Input: part model. Units: mm. Frame: model coordinates. A direction names the side the tool comes from. Round coordinates to 2 decimals unless told otherwise and drop trailing zeros. Write each loop counter-clockwise with the first axis right and the second up, starting at its lowest first coordinate (ties: lowest second). Pieces come first, ordered by that corner, then holes. Notation, with made-up numbers: (17.5, 40) - (39.5, 40) arc R13 cw to (39.5, 62) - close; hole circle Ø1 at (-15.75, 80.5). An arc over 180 degrees is marked (long way). One line per item, written item: value. Start each with the question number.
```python
from build123d import *

# Parameters (mm, degrees)
BOSS_EXTRUDE1_DEPTH = 4
CHAMFER1_SIZE       = 0.4
BOSS_EXTRUDE2_START = 4
SKETCH3_R           = 2.5
BOSS_EXTRUDE2_DEPTH = 0.01


with BuildPart() as part:
    # Sketch1 → Boss-Extrude1 (new body)
    with BuildSketch(Plane(origin=(0, 0, 0), x_dir=(1, 0, 0), z_dir=(0, 1, 0))):
        with BuildLine():
            Line((-12.75, -10.75), (9.25, -10.75))
            ThreePointArc((9.25, -10.75), (10.310660172, -10.310660172), (10.75, -9.25))
            Line((10.75, -9.25), (10.75, 12.75))
            ThreePointArc((10.75, 12.75), (10.310660172, 13.810660172), (9.25, 14.25))
            Line((9.25, 14.25), (-11.25, 14.25))
            ThreePointArc((-11.25, 14.25), (-13.371320344, 13.371320344), (-14.25, 11.25))
            Line((-14.25, 11.25), (-14.25, -9.25))
            ThreePointArc((-14.25, -9.25), (-13.810660172, -10.310660172), (-12.75, -10.75))
        make_face()
    extrude(amount=BOSS_EXTRUDE1_DEPTH)

    # Chamfer1
    chamfer1_edges = [part.edges().sort_by_distance(p)[0] for p in [
        (-13.810660172, 4, 10.310660172),
        (-14.25, 0, -1),
        (-13.371320344, 0, -13.371320344),
        (-1.75, 4, 10.75),
        (10.310660172, 4, 10.310660172),
        (10.75, 4, -1.75),
        (10.310660172, 4, -13.810660172),
        (-1, 4, -14.25),
        (-13.371320344, 4, -13.371320344),
        (-14.25, 4, -1),
        (-1, 0, -14.25),
        (10.310660172, 0, -13.810660172),
        (10.75, 0, -1.75),
        (10.310660172, 0, 10.310660172),
        (-1.75, 0, 10.75),
        (-13.810660172, 0, 10.310660172),
    ]]
    chamfer(chamfer1_edges, length=CHAMFER1_SIZE)

    # Sketch2 → Revolve1 (revolve)
    with BuildSketch(Plane.XY):
        with BuildLine():
            Line((-3.215339078, 1.983898683), (-0.5, 1.983898683))
            Line((-0.5, 1.983898683), (-0.5, -2.4))
            Line((-0.5, -2.4), (0, -2.4))
            Line((0, -2.4), (0, 4.5))
            ThreePointArc((0, 4.5), (-2.041394819, 3.796209153), (-3.215339078, 1.983898683))
        make_face()
    revolve(axis=Axis((0, 5.892068095, 0), (0, -1, 0)))

    # Sketch3 → Boss-Extrude2 (add)
    with BuildSketch(Plane(origin=(0, 0, 0), x_dir=(1, 0, 0), z_dir=(0, 1, 0)).offset(BOSS_EXTRUDE2_START)):
        Polygon((-10.25, 11.25), (7.75, 11.25), (8.75, 10.25), (8.75, 3.25), (9.25, 3.25), (9.25, -0.75), (8.75, -0.75), (8.75, -7.75), (7.75, -8.75), (-10.25, -8.75), (-11.25, -7.75), (-11.25, -0.75), (-11.75, -0.75), (-11.75, 3.25), (-11.25, 3.25), (-11.25, 10.25), align=None)
        Circle(SKETCH3_R, mode=Mode.SUBTRACT)
    extrude(amount=BOSS_EXTRUDE2_DEPTH)


solid = part.part
```
Q1. Contact query for flat-ended pins moving along their axis: pin 1 Ø1 at (x, z) = (1, 4.5) entering from +Y; pin 2 Ø4 at (x, z) = (-7.5, -3.5) entering from -Y. Output: stop coordinate, or through.
Q2. Cut plane C-C, the plane y = -0.75. Output: boundary loops of the cut face in (x, z).
Q3. Access query for faces 1 (the conical face through (10.126, 3.847, 10.146)), 2 (the cylindrical face through (0.108, -1.217, 0.488)). Directions: +Z, -Z, +X, -X, +Y, -Y. A direction counts if a zero-diameter tool reaches every point of the face in a straight line with its end or side. Return the directions, or none.
Q4. Material intervals for probe 1 along Y at (x, z) = (-2.25, 1.5); probe 2 along X at (y, z) = (3.75, -9.25); probe 3 along X at (y, z) = (4.05, 0), sorted ascending. Write a range as from..to.
A:
1. pin 1: stops at y = 4.01
1. pin 2: stops at y = 0
2. outline: circle Ø1 at (0, 0)
3. face 1: +Z, +X, +Y
3. face 2: -Y
4. probe 1: y = 0..4.01
4. probe 2: x = -14.1..10.6
4. probe 3: x = -1.67..1.67
